```python
from build123d import *

# Parameters (mm, degrees)
CUT_EXTRUDE_1_DEPTH = 4
FILLET_1_R          = 1
FILLET_2_R          = 0.2


with BuildPart() as part:
    # Эскиз1 → Повернуть1 (revolve)
    with BuildSketch(Plane.XY):
        Polygon((-8, 0), (-8, 6.5), (0, 6.5), (0, 4), (16, 4), (16, 0), align=None)
    revolve(axis=Axis((-351.589582302, 0, 0), (1, 0, 0)))

    # Эскиз2 → Вырез-Вытянуть1 (cut)
    with BuildSketch(Plane.ZY.offset(8)):
        Polygon((0, -3.464101615), (3, -1.732050808), (3, 1.732050808), (0, 3.464101615), (-3, 1.732050808), (-3, -1.732050808), align=None)
    extrude(amount=-CUT_EXTRUDE_1_DEPTH, mode=Mode.SUBTRACT)

    # Скругление1
    fillet_1_edges = [part.edges().sort_by_distance(p)[0] for p in [
        (-8, -6.5, 0),
    ]]
    fillet(fillet_1_edges, radius=FILLET_1_R)

    # Скругление2
    fillet_2_edges = [part.edges().sort_by_distance(p)[0] for p in [
        (-8, -2.598076211, -1.5),
        (-8, -2.598076211, 1.5),
        (-8, 0, 3),
        (-8, 2.598076211, 1.5),
        (-8, 2.598076211, -1.5),
        (-8, 0, -3),
    ]]
    fillet(fillet_2_edges, radius=FILLET_2_R)


solid = part.part
```
Geometry: final body of the model. Coordinates: model frame, mm. A direction names the side the tool comes from. Round coordinates to 2 decimals unless told otherwise and drop trailing zeros. Loops run counter-clockwise (first coordinate to the right, second up) from the corner with the lowest first, then second, coordinate; pieces in that order, holes last.
Item 1: Mould query, pull axis Z, two halves, no side actions, for faces 1 (the cylindrical face through (8.112, -0.867, -3.905)), 2 (the cylindrical face through (-7.943, -2.637, 1.552)), 3 (the flat face through (16, 0, 0)). Classes: released by +Z, released by -Z, zero draft, split by the parting line, or undercut.
Checked values:
face 1: split by the parting line
face 2: undercut
face 3: zero draft
Item 2: Section C-C, the plane x = 13. Output: boundary loops of the cut face in (y, z), plus the area to 3 significant figures.
Checked values:
outline: circle Ø8 at (0, 0)
area: 50.3 mm2
Item 3: Reachability of faces 4 (the flat face through (0, 3, 3)), 5 (the cylindrical face through (-3.451, -5.158, -3.955)), 6 (the cylindrical face through (-7.94, 2.66, 1.51)) from +Z, -Z, +X, -X, +Y, -Y: full face, straight path, thin tool, end or side. Return the list, or none.
Checked values:
face 4: +X
face 5: +X, -X
face 6: -X
Item 4: Section B-B, the plane x = -2. Output: boundary loops of the cut face in (y, z).
Checked values:
outline: circle Ø13 at (0, 0)
Item 5: Section A-A, the plane y = 0. Output: boundary loops of the cut face in (x, z).
Checked values:
outline: (-8, -5.5) arc R1 ccw to (-7, -6.5) - (0, -6.5) - (0, -4) - (16, -4) - (16, 4) - (0, 4) - (0, 6.5) - (-7, 6.5) arc R1 ccw to (-8, 5.5) - (-8, 3.2) arc R0.2 ccw to (-7.8, 3) - (-4, 3) - (-4, -3) - (-7.8, -3) arc R0.2 ccw to (-8, -3.2) - close
Item 6: Line query: L1, parallel to X at y = 4.25, z = -1; L2, parallel to Y at x = 7, z = 2; L3, parallel to X at y = 2.75, z = 1. Output: solid intervals per line, ascending.
Checked values:
L1: x = -8 to 0
L2: y = -3.46 to 3.46
L3: x = -4 to 16
Item 7: Contact query for flat-ended pins moving along their axis: P1, Ø1, axis at x = 7, z = -2, coming from the +Y side; P2, Ø1, axis at x = 2, z = 4, coming from the -Y side; P3, Ø2, axis at x = -4.5, y = -1.5, coming from the +Z side. Output: stop coordinate, or through.
Checked values:
P1: stops at y = 3.71
P2: stops at y = -1.94
P3: stops at z = 6.48
